from build123d import *

# Parameters (mm, degrees)
BOSS_EXTRU_1_DEPTH = 80
BOSS_EXTRU_3_DEPTH = 80


with BuildPart() as part:
    # Esquisse1 → Boss.-Extru.1 (new body)
    with BuildSketch(Plane.XY):
        Polygon((0, 0), (0, 80), (120, 80), (120, 70), (23, 70), (23, 0), (13, 0), (13, 70), (7, 70), (7, 0), align=None)
    extrude(amount=BOSS_EXTRU_1_DEPTH)

    # Esquisse2 → Boss.-Extru.3 (add)
    with BuildSketch(Plane(origin=(0, 0, 0), x_dir=(-1, 0, 0), z_dir=(0, 0, -1))):
        Polygon((-71.5, 70), (-23, 35), (-23, 22.668017278), (-88.588604629, 70), align=None)
    extrude(amount=-BOSS_EXTRU_3_DEPTH)


solid = part.part
Could you check a few things on this model? Use its own coordinates, in mm. A direction names the side the tool comes from. Coordinates: 2 decimals unless noted, no trailing zeros. Order: outer loops, then holes, each group sorted by start corner. A loop starts at its lowest first (then second) coordinate and runs counter-clockwise, first axis right, second up.
Q1. Suppose I cut it at D-D on y = 60.5. Please give me the cut outline in (x, z), and give its area (3 significant figures).
Q2. Suppose I cut it at A-A on y = 15. Please give me the cut outline in (x, z).
Q3. Thinking about a two-plate mould opening in Y: for faces 6 (the flat face through (7, 35, 39)), 7 (the flat face through (18, 0, 39)), 8 (the flat face through (48, 70, 39)), which applies, released by +Y, released by -Y, zero draft, split by the parting line, or undercut?
Q4. Suppose I cut it at B-B on z = 24. Please give me the cut outline in (x, y), and give its area (3 significant figures).
Q5. Which directions (+Z, -Z, +X, -X, +Y, -Y) give clear straight access to the entire face, cutting with the end or side of a thin tool? Please do faces 1 (the flat face through (38, 43, 80)), 2 (the flat face through (10, 70, 39)), 3 (the flat face through (23, 53, 39)), 4 (the flat face through (120, 75, 39)), 5 (the flat face through (105, 70, 39)).
Q6. Please list where these lines run through material, in increasing order: L1, parallel to X at y = 55, z = 12.5; L2, parallel to X at y = 43.5, z = 38; L3, parallel to Y at x = 108, z = 5.
Q7. Will these pins go through, and if not, where does the flat tip stop? pin 1 (21 mm diameter, centred on y = 45.5, z = 46, fed in from +X); pin 2 (24 mm diameter, centred on x = 54, z = 34, fed in from -Y); pin 3 (5 mm diameter, centred on x = 75, z = 20, fed in from -Y); pin 4 (12 mm diameter, centred on y = 60, z = 56, fed in from -X).
Q8. Suppose I cut it at C-C on x = 52.5. Please give me the cut outline in (y, z).
Answer:
1. outline: (0, 0) - (7, 0) - (7, 80) - (0, 80) - close; (13, 0) - (23, 0) - (23, 80) - (13, 80) - close; (58.34, 0) - (75.42, 0) - (75.42, 80) - (58.34, 80) - close
1. area: 2,730 mm2
2. outline: (0, 0) - (7, 0) - (7, 80) - (0, 80) - close; (13, 0) - (23, 0) - (23, 80) - (13, 80) - close
3. face 6: zero draft
3. face 7: released by -Y
3. face 8: undercut
4. outline: (0, 0) - (7, 0) - (7, 70) - (13, 70) - (13, 0) - (23, 0) - (23, 22.67) - (88.59, 70) - (120, 70) - (120, 80) - (0, 80) - close; hole (23, 35) - (71.5, 70) - (23, 70) - close
4. area: 3,090 mm2
5. face 1: +Z, +X, -X, +Y, -Y
5. face 2: +Z, -Z, -Y
5. face 3: +Z, -Z
5. face 4: +Z, -Z, +X, +Y, -Y
5. face 5: +Z, -Z, +X, -Y
6. L1: x = 0 to 7, 13 to 23, 50.71 to 67.8
6. L2: x = 0 to 7, 13 to 23, 34.78 to 51.87
6. L3: y = 70 to 80
7. pin 1: stops at x = 69.19
7. pin 2: stops at y = 36.38
7. pin 3: stops at y = 58.39
7. pin 4: stops at x = 0
8. outline: (43.96, 0) - (56.29, 0) - (56.29, 80) - (43.96, 80) - close; (70, 0) - (80, 0) - (80, 80) - (70, 80) - close
